Geometry: see drawing. Coordinates: mm, zero at the bounding-box minimum. A direction names the side the tool comes from. Give positions to 0.01 mm unless a question says otherwise; leave off trailing zeros. Write each loop counter-clockwise with the first axis right and the second up, starting at its lowest first coordinate (ties: lowest second). Pieces come first, ordered by that corner, then holes. Notation, with made-up numbers: (42, 2) - (95, 2) arc R24 ccw to (95, 19) - close; hole circle Ø1 at (-29, 76.25). An arc over 180 degrees is marked (long way). Answer as CSV lines item,"result". Start each with the question number.
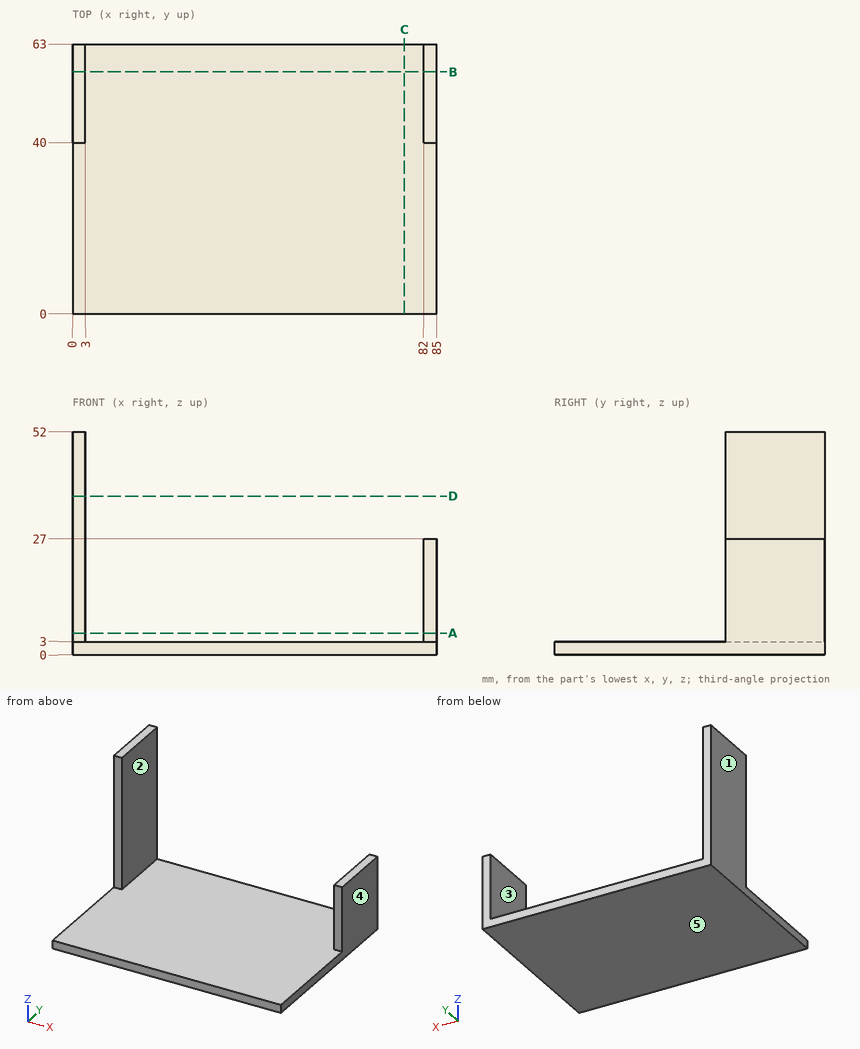
1) Cut plane D-D on z = 37. Output: boundary loops of the cut face in (x, y).
2) Contact query for flat-ended pins moving along their axis: P1, Ø4, axis at x = 64.5, y = 45.5, coming from the +Z side; P2, Ø1.5, axis at x = 2, z = 20, coming from the -Y side; P3, Ø4, axis at y = 44.5, z = 32.5, coming from the +X side. Output: stop coordinate, or through.
3) Cut plane A-A on z = 5. Output: boundary loops of the cut face in (x, y).
4) Pull-direction query (X, two-part tool) for the marked faces 3, 4 and 5; classes: +X half, -X half, draft (parallel to the pull), parting line (faces both ways), or undercut.
5) Material intervals for line 1 (X direction, y = 50, z = 18); line 2 (Z direction, x = 38, y = 41), sorted ascending. Write a range as from..to.
6) Cut plane C-C on x = 77.5. Output: boundary loops of the cut face in (y, z), and give its area (3 significant figures).
7) Cut plane B-B on y = 56.5. Output: boundary loops of the cut face in (x, z).
8) Reachability of the marked faces 1 and 2 from +Z, -Z, +X, -X, +Y, -Y: full face, straight path, thin tool, end or side. Return the list, or none.
Numbers:
1,outline,"(0, 40) - (3, 40) - (3, 63) - (0, 63) - close"
2,P1,"stops at z = 3"
2,P2,"stops at y = 40"
2,P3,"stops at x = 3"
3,outline,"(0, 40) - (3, 40) - (3, 63) - (0, 63) - close; (82, 40) - (85, 40) - (85, 63) - (82, 63) - close"
4,face 3,"undercut"
4,face 4,"+X half"
4,face 5,"draft"
5,line 1,"x = 0..3, 82..85"
5,line 2,"z = 0..3"
6,outline,"(0, 0) - (63, 0) - (63, 3) - (0, 3) - close"
6,area,"189 mm²"
7,outline,"(0, 0) - (85, 0) - (85, 27) - (82, 27) - (82, 3) - (3, 3) - (3, 52) - (0, 52) - close"
8,face 1,"+Z, -Z, -X, +Y, -Y"
8,face 2,"+Z, +Y, -Y"
